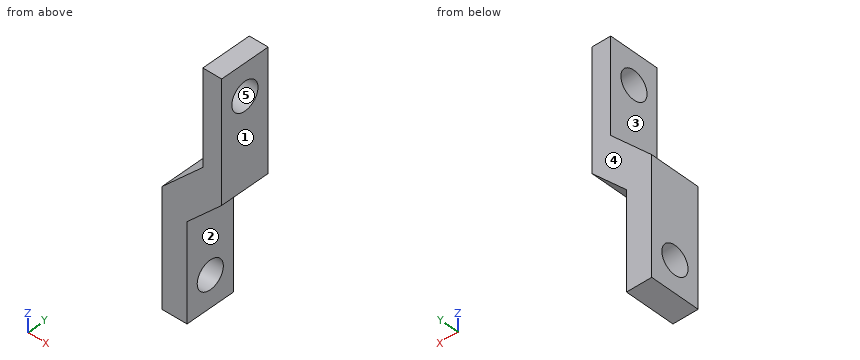
from build123d import *

# Parameters (mm, degrees)
BOSS_EXTRUDE1_DEPTH     = 8
SKETCH2_R               = 2.25
CUT_EXTRUDE1_DEPTH      = 6.5
CUT_EXTRUDE1_DEPTH_BACK = 5


with BuildPart() as part:
    # Sketch1 → Boss-Extrude1 (new body)
    with BuildSketch(Plane(origin=(0, 0, 0), x_dir=(1, 0, 0), z_dir=(0, 1, 0))):
        Polygon((0, 0), (-3, 0), (-3, 15), (-9.5, 21.5), (-9.5, 40), (-5.5, 40), (-5.5, 24.571067812), (0, 19.071067812), align=None)
    extrude(amount=BOSS_EXTRUDE1_DEPTH)

    # Sketch2 → Cut-Extrude1 (cut, two sides)
    with BuildSketch(Plane(origin=(-5.5, 0, 0), x_dir=(0, 0, -1), z_dir=(1, 0, 0))) as cut_extrude1_sk:
        with Locations((35, 4)):
            Circle(SKETCH2_R)
        with Locations((5, 4)):
            Circle(SKETCH2_R)
    extrude(amount=CUT_EXTRUDE1_DEPTH, mode=Mode.SUBTRACT)
    extrude(cut_extrude1_sk.sketch, amount=-CUT_EXTRUDE1_DEPTH_BACK, mode=Mode.SUBTRACT)


solid = part.part
Here's how the part is built. I have some questions about the finished solid (model axes, mm). Face numbers are marked on the shaded views. A direction names the side the tool comes from. Coordinates: 2 decimals unless noted, no trailing zeros. Write each loop counter-clockwise with the first axis right and the second up, starting at its lowest first coordinate (ties: lowest second). Pieces come first, ordered by that corner, then holes.
1) I'm going to push flat-ended pins straight in: pin 1 (2 mm diameter, centred on x = -3.5, y = 1.5, fed in from -Z); pin 2 (2 mm diameter, centred on y = 3, z = -22, fed in from +X); pin 3 (2.5 mm diameter, centred on y = 5.5, z = -31.5, fed in from +X). Where does each tip first touch, or does it pass through?
Filled in:
pin 1: stops at z = -23.57
pin 2: stops at x = -1.93
pin 3: stops at x = -5.5
2) If we section it at D-D (z = -5): List the corners of the cut face in (x, y) for me.
Filled in:
outline: (-3, 0) - (0, 0) - (0, 1.75) - (-3, 1.75) - close; (-3, 6.25) - (0, 6.25) - (0, 8) - (-3, 8) - close
3) If we section it at C-C (x = -6.5): List the corners of the cut face in (y, z) for me.
Filled in:
outline: (0, -40) - (8, -40) - (8, -18.5) - (0, -18.5) - close; hole circle Ø4.5 at (4, -35)
4) Thinking about a two-plate mould opening in Y: for the marked faces 3, 4 and 5, which applies, +Y half, -Y half, draft (parallel to the pull), parting line (faces both ways), or undercut?
Filled in:
face 3: draft
face 4: +Y half
face 5: undercut
5) If we section it at A-A (y = 4): List the corners of the cut face in (x, z) for me, plus the area to 3 significant figures.
Filled in:
outline: (-9.5, -40) - (-5.5, -40) - (-5.5, -37.25) - (-9.5, -37.25) - close; (-9.5, -32.75) - (-5.5, -32.75) - (-5.5, -24.57) - (0, -19.07) - (0, -7.25) - (-3, -7.25) - (-3, -15) - (-9.5, -21.5) - close; (-3, -2.75) - (0, -2.75) - (0, 0) - (-3, 0) - close
area: 130 mm2
6) If I drill on line 1 (X direction, y = 2.5, z = -8); line 2 (X direction, y = 0.5, z = -32.5); line 3 (Y direction, x = -6.25, z = -35), over which ranges is the centre line in solid material (lowest first)?
Filled in:
line 1: x = -3 to 0
line 2: x = -9.5 to -5.5
line 3: y = 0 to 1.75, 6.25 to 8
7) Which directions (+Z, -Z, +X, -X, +Y, -Y) give clear straight access to the entire face, cutting with the end or side of a thin tool? Please do the marked faces 1 and 2.
Filled in:
face 1: +Z, -Z, +X, +Y, -Y
face 2: -Z, +X, +Y, -Y
8) If we section it at B-B (z = -35): List the corners of the cut face in (x, y) for me.
Filled in:
outline: (-9.5, 0) - (-5.5, 0) - (-5.5, 1.75) - (-9.5, 1.75) - close; (-9.5, 6.25) - (-5.5, 6.25) - (-5.5, 8) - (-9.5, 8) - close
